Part model, mm, in its own coordinate system. A direction names the side the tool comes from. Give positions to 0.01 mm unless a question says otherwise; leave off trailing zeros. Loops run counter-clockwise (first coordinate to the right, second up) from the corner with the lowest first, then second, coordinate; pieces in that order, holes last. Notation, with made-up numbers: M 35,87 L 47,87 A15 ccw 47,98 Z; hole C 13,76 d11. An arc over 180 degrees is marked long. Answer in a Markdown table with one row per item.
from build123d import *

# Parameters (mm, degrees)
SKETCH_1_W          = 66
SKETCH_1_H          = 36
SKETCH_1_R          = 1.75
EXTRUDE_1_DEPTH     = 2
SKETCH_2_W          = 22
SKETCH_2_H          = 14
EXTRUDE_2_DEPTH     = 7
SKETCH_3_W          = 5
SKETCH_3_H          = 10
EXTRUDE_3_DEPTH     = 10
CUT_EXTRUDE_1_DEPTH = 0.2
SKETCH_5_R          = 1.5
SKETCH_5_R_2        = 1
CUT_EXTRUDE_2_DEPTH = 0.2


with BuildPart() as part:
    # 草图1 → 凸台-拉伸1 (new body)
    with BuildSketch(Plane.XY):
        Rectangle(SKETCH_1_W, SKETCH_1_H)
        with Locations((30.5, 15.5)):
            Circle(SKETCH_1_R, mode=Mode.SUBTRACT)
        with Locations(Location((30.5, -15.5, 0), (0, 0, 180))):
            Circle(SKETCH_1_R, mode=Mode.SUBTRACT)
        with Locations((-30.5, -15.5)):
            Circle(SKETCH_1_R, mode=Mode.SUBTRACT)
        with Locations(Location((-30.5, 15.5, 0), (0, 0, 180))):
            Circle(SKETCH_1_R, mode=Mode.SUBTRACT)
    extrude(amount=EXTRUDE_1_DEPTH)

    # 草图2 → 凸台-拉伸2 (add)
    with BuildSketch(Plane.XY.offset(2)):
        with Locations((0, -10.8)):
            Rectangle(SKETCH_2_W, SKETCH_2_H)
    extrude(amount=EXTRUDE_2_DEPTH)

    # 草图3 → 凸台-拉伸3 (add)
    with BuildSketch(Plane.XY.offset(2)):
        with Locations((-30.5, 0)):
            Rectangle(SKETCH_3_W, SKETCH_3_H)
        with Locations((30.5, 0)):
            Rectangle(SKETCH_3_W, SKETCH_3_H)
    extrude(amount=EXTRUDE_3_DEPTH)

    # 草图4 → 切除-拉伸1 (cut)
    with BuildSketch(Plane.XY.offset(12)):
        Polygon((29, 0.571414009), (29, -0.928585991), (29.5, -0.928585991), (29.5, -0.428585991), (31.5, -0.428585991), (31.5, -0.928585991), (32, -0.928585991), (32, 0.571414009), (31.5, 0.571414009), (31.5, 0.071414009), (29.5, 0.071414009), (29.5, 0.571414009), align=None)
    extrude(amount=-CUT_EXTRUDE_1_DEPTH, mode=Mode.SUBTRACT)

    # 草图5 → 切除-拉伸2 (cut)
    with BuildSketch(Plane.XY.offset(12)):
        with Locations((-30.551618455, 0)):
            Circle(SKETCH_5_R)
        with Locations((-30.551618455, 0)):
            Circle(SKETCH_5_R_2, mode=Mode.SUBTRACT)
    extrude(amount=-CUT_EXTRUDE_2_DEPTH, mode=Mode.SUBTRACT)


solid = part.part
(1) Saw through at D-D (z = 7.5). Write the cut outline in (x, y), plus the area to 3 significant figures.
Recorded:
| item | result |
|---|---|
| outline | M -33,-5 L -28,-5 L -28,5 L -33,5 Z; M -11,-17.8 L 11,-17.8 L 11,-3.8 L -11,-3.8 Z; M 28,-5 L 33,-5 L 33,5 L 28,5 Z |
| area | 408 mm^2 |
(2) Pin check, flat tips, straight feed: pin 1 Ø4 at (x, z) = (-31.5, 7) entering from -Y; pin 2 Ø4 at (y, z) = (-10, 5.5) entering from +X; pin 3 Ø2 at (x, y) = (-30.5, -15.5) entering from +Z; pin 4 Ø1.5 at (x, y) = (4, 4) entering from +Z. Stop position of each tip, or through.
Recorded:
| item | result |
|---|---|
| pin 1 | stops at y = -5 |
| pin 2 | stops at x = 11 |
| pin 3 | passes through |
| pin 4 | stops at z = 2 |
(3) Pull direction Y, two halves, no side cores. Call faces 5 (the face through (33, 0, 5)), 6 (the face through (-31.79, -14.32, 0.99)), 7 (the face through (30, 5, 7)): +Y half, -Y half, draft (parallel to the pull), parting line (faces both ways), or undercut.
Recorded:
| item | result |
|---|---|
| face 5 | draft |
| face 6 | undercut |
| face 7 | +Y half |
(4) Which spindle directions (+Z, -Z, +X, -X, +Y, -Y) get a long thin tool onto all of the face, cutting with end or side? Do faces 1 (the face through (-31, -5, 7)), 2 (the face through (30, -5, 7)), 3 (the face through (0, -17.8, 5)), 4 (the face through (0, -3.8, 5)). Say none if no direction does.
Recorded:
| item | result |
|---|---|
| face 1 | +Z, -X, -Y |
| face 2 | +Z, +X, -Y |
| face 3 | +Z, +X, -X, -Y |
| face 4 | +Z, +Y |
(5) Saw through at C-C (z = 10.25). Write the cut outline in (x, y), plus the area to 3 significant figures.
Recorded:
| item | result |
|---|---|
| outline | M -33,-5 L -28,-5 L -28,5 L -33,5 Z; M 28,-5 L 33,-5 L 33,5 L 28,5 Z |
| area | 100 mm^2 |
(6) Saw through at B-B (x = 30.5). Write the cut outline in (y, z).
Recorded:
| item | result |
|---|---|
| outline | M -18,0 L -17.25,0 L -17.25,2 L -18,2 Z; M -13.75,0 L 13.75,0 L 13.75,2 L 5,2 L 5,12 L 0.07,12 L 0.07,11.8 L -0.43,11.8 L -0.43,12 L -5,12 L -5,2 L -13.75,2 Z; M 17.25,0 L 18,0 L 18,2 L 17.25,2 Z |
(7) Saw through at A-A (y = -15.5). Write the cut outline in (x, z), plus the area to 3 significant figures.
Recorded:
| item | result |
|---|---|
| outline | M -33,0 L -32.25,0 L -32.25,2 L -33,2 Z; M -28.75,0 L 28.75,0 L 28.75,2 L 11,2 L 11,9 L -11,9 L -11,2 L -28.75,2 Z; M 32.25,0 L 33,0 L 33,2 L 32.25,2 Z |
| area | 272 mm^2 |
(8) Drill centre lines: line 1 along Y through (x, z) = (30.5, 0.5); line 2 along X through (y, z) = (2, 6.25); line 3 along X through (y, z) = (16, 1.75). Where is each one in solid material? Low to high.
Recorded:
| item | result |
|---|---|
| line 1 | y = -18 to -17.25, -13.75 to 13.75, 17.25 to 18 |
| line 2 | x = -33 to -28, 28 to 33 |
| line 3 | x = -33 to -32.18, -28.82 to 28.82, 32.18 to 33 |
